```python
from build123d import *

# Parameters (mm, degrees)
SKETCH_1_W          = 25
SKETCH_1_H          = 25
EXTRUDE_1_DEPTH     = 3
FILLET_1_R          = 8
FILLET_2_R          = 8
FILLET_3_R          = 8
SKETCH_2_R          = 4.1
CUT_EXTRUDE_1_DEPTH = 3
CUT_EXTRUDE_2_DEPTH = 3


with BuildPart() as part:
    # 草图1 → 凸台-拉伸1 (new body)
    with BuildSketch(Plane.XY):
        Rectangle(SKETCH_1_W, SKETCH_1_H)
    extrude(amount=EXTRUDE_1_DEPTH)

    # 圆角1
    fillet_1_edges = [part.edges().sort_by_distance(p)[0] for p in [
        (-12.5, -12.5, 1.5),
    ]]
    fillet(fillet_1_edges, radius=FILLET_1_R)

    # 圆角2
    fillet_2_edges = [part.edges().sort_by_distance(p)[0] for p in [
        (12.5, -12.5, 1.5),
    ]]
    fillet(fillet_2_edges, radius=FILLET_2_R)

    # 圆角3
    fillet_3_edges = [part.edges().sort_by_distance(p)[0] for p in [
        (12.5, 12.5, 1.5),
    ]]
    fillet(fillet_3_edges, radius=FILLET_3_R)

    # 草图2 → 切除-拉伸1 (cut)
    with BuildSketch(Plane.XY.offset(3)):
        with Locations((4.1, -4.1)):
            Circle(SKETCH_2_R)
    extrude(amount=-CUT_EXTRUDE_1_DEPTH, mode=Mode.SUBTRACT)

    # 草图3 → 切除-拉伸2 (cut)
    with BuildSketch(Plane.XY.offset(3)):
        with BuildLine():
            Line((12.256606279, -6.458330674), (6.999137803, -1.200862197))
            ThreePointArc((6.999137803, -1.200862197), (6.999137803, -6.999137803), (1.200862197, -6.999137803))
            Line((1.200862197, -6.999137803), (6.458330674, -12.256606279))
            ThreePointArc((6.458330674, -12.256606279), (10.156854249, -10.156854249), (12.256606279, -6.458330674))
        make_face()
    extrude(amount=-CUT_EXTRUDE_2_DEPTH, mode=Mode.SUBTRACT)


solid = part.part
```
The model under review builds one solid part; all positions refer to its coordinate system, in mm. A direction names the side the tool comes from. Give positions to 0.01 mm unless a question says otherwise; leave off trailing zeros. Write each loop counter-clockwise with the first axis right and the second up, starting at its lowest first coordinate (ties: lowest second). Pieces come first, ordered by that corner, then holes. Notation, with made-up numbers: (71, -3.5) -> (130, -3.5) arc R27 cw to (130, 33.5) -> close; hole circle Ø5 at (32, 17.25). An arc over 180 degrees is marked (long way). Put each result on its own line as item: value.
(1) We need section C-C, the plane z = 1.85. Give the boundary of the cut face in (x, y).
Results are:
outline: (-12.5, -4.5) arc R8 ccw to (-4.5, -12.5) -> (4.5, -12.5) arc R8 ccw to (6.46, -12.26) -> (1.2, -7) arc R4.1 cw to (7, -1.2) -> (12.26, -6.46) arc R8 ccw to (12.5, -4.5) -> (12.5, 4.5) arc R8 ccw to (4.5, 12.5) -> (-12.5, 12.5) -> close
(2) We need section A-A, the plane y = -5.5. Give the boundary of the cut face in (x, z).
Results are:
outline: (-12.44, 0) -> (0.25, 0) -> (0.25, 3) -> (-12.44, 3) -> close; (11.3, 0) -> (12.44, 0) -> (12.44, 3) -> (11.3, 3) -> close
(3) We need section D-D, the plane y = 8. Give the boundary of the cut face in (x, z), and give its area (3 significant figures).
Results are:
outline: (-12.5, 0) -> (11.69, 0) -> (11.69, 3) -> (-12.5, 3) -> close
area: 72.6 mm²
(4) To check wall thickness, follow probe 1 along X at (y, z) = (-1, 2.35); probe 2 along Y at (x, z) = (3.25, 1.75); probe 3 along X at (y, z) = (-4.5, 0.9). State the ranges of each line that lie inside material, in increasing order. Write a range as from..to.
Results are:
probe 1: -12.5..1.42, 6.78..12.5
probe 2: -12.5..-9.05, -0.09..12.5
probe 3: -12.5..0.02, 10.3..12.5
(5) Tool access review of faces 4 (the flat face through (3.8, -9.6, 1.5)), 5 (the flat face through (9.7, -3.9, 1.5)), 6 (the flat face through (-12.5, 4, 1)): name each direction out of +Z, -Z, +X, -X, +Y, -Y from which nothing blocks a thin tool from reaching the whole face with its end or side.
Results are:
face 4: +Z, -Z, +X
face 5: +Z, -Z, -Y
face 6: +Z, -Z, -X, +Y, -Y
(6) The part is to be moulded in two halves that separate along Z. For faces 1 (the flat face through (-3, 3, 3)), 2 (the flat face through (0, -12.5, 1)), 3 (the flat face through (-3, 3, 0)), say which applies: pulls with the +Z half, pulls with the -Z half, needs draft (parallel to the pull), parting line crosses it, or undercut.
Results are:
face 1: pulls with the +Z half
face 2: needs draft
face 3: pulls with the -Z half
(7) We need section B-B, the plane x = 4.1. Give the boundary of the cut face in (y, z).
Results are:
outline: (-12.5, 0) -> (-9.9, 0) -> (-9.9, 3) -> (-12.5, 3) -> close; (0, 0) -> (12.5, 0) -> (12.5, 3) -> (0, 3) -> close
